Autodesk Inventor part; units mm, degrees
ref_plane "YZ Plane" through (0, 0, 0) normal (1, 0, 0) x (0, 1, 0)
ref_plane "XZ Plane" through (0, 0, 0) normal (0, 1, 0) x (-1, 0, 0)
ref_plane "XY Plane" through (0, 0, 0) normal (0, 0, 1) x (1, 0, 0)
sketch "T-Slot 4040 Base" plane through (0, 0, 0) normal (0, 0, 1) x (1, 0, 0)
  line L0 (-28, 0) -> (28, 0) construction
  line L1 (0, -28) -> (0, 28) construction
  circle A0 centre (0, 0) radius 5.1
  line L2 (-7.5, -7.5) -> (7.5, -7.5)
  line L3 (7.5, -7.5) -> (7.5, 7.5)
  line L4 (7.5, 7.5) -> (-7.5, 7.5)
  line L5 (-7.5, 7.5) -> (-7.5, -7.5)
  line L6 (-7.5, -7.5) -> (7.5, 7.5) construction
  line L7 (7.5, -7.5) -> (-7.5, 7.5) construction
  line L8 (-20, 20) -> (20, 20)
  line L9 (20, 20) -> (20, -20)
  line L10 (20, -20) -> (-20, -20)
  line L11 (-20, -20) -> (-20, 20)
  line L12 (-20, 20) -> (20, -20) construction
  line L13 (20, 20) -> (-20, -20) construction
  line L14 (20, 5) -> (14.5, 5)
  line L15 (14.5, 5) -> (14.5, 10)
  line L16 (14.5, 10) -> (12.4749, 10)
  line L17 (12.4749, 10) -> (7.5, 5.0251)
  line L18 (5, 20) -> (5, 14.5)
  line L19 (5, 14.5) -> (10, 14.5)
  line L20 (10, 14.5) -> (10, 12.4749)
  line L21 (10, 12.4749) -> (5.0251, 7.5)
  line L22 (18.5, 18.5) -> (11.5, 18.5)
  line L23 (11.5, 18.5) -> (11.5, 11.5)
  line L24 (11.5, 11.5) -> (18.5, 11.5)
  line L25 (18.5, 11.5) -> (18.5, 18.5)
  line L26 (18.5, 18.5) -> (11.5, 11.5) construction
  line L27 (11.5, 18.5) -> (18.5, 11.5) construction
  line L28 (3.0732, 1.3088) -> (4.38, 2.6125) construction
  line L29 (5.905, 4.1338) -> (4.1393, 5.9037)
  line L30 (4.1393, 5.9037) -> (2.6122, 4.3802)
  line L31 (1.3075, 3.0787) -> (3.0732, 1.3088) construction
  line L32 (3.0732, 1.3088) -> (4.1393, 5.9037) construction
  line L33 (5.905, 4.1338) -> (1.3075, 3.0787) construction
  line L34 (4.38, 2.6125) -> (5.905, 4.1338)
  line L35 (2.6122, 4.3802) -> (1.3075, 3.0787) construction
  line L36 (-20, 5) -> (-14.5, 5)
  line L37 (-14.5, 5) -> (-14.5, 10)
  line L38 (-14.5, 10) -> (-12.4749, 10)
  line L39 (-12.4749, 10) -> (-7.5, 5.0251)
  line L40 (-5, 20) -> (-5, 14.5)
  line L41 (-5, 14.5) -> (-10, 14.5)
  line L42 (-10, 14.5) -> (-10, 12.4749)
  line L43 (-10, 12.4749) -> (-5.0251, 7.5)
  line L44 (-18.5, 18.5) -> (-11.5, 18.5)
  line L45 (-11.5, 18.5) -> (-11.5, 11.5)
  line L46 (-11.5, 11.5) -> (-18.5, 11.5)
  line L47 (-18.5, 11.5) -> (-18.5, 18.5)
  line L48 (-5.905, 4.1338) -> (-4.1393, 5.9037)
  line L49 (-4.1393, 5.9037) -> (-2.6122, 4.3802)
  line L50 (-4.38, 2.6125) -> (-5.905, 4.1338)
  line L51 (7.5, -7.5) -> (-7.5, -7.5)
  line L52 (20, -5) -> (14.5, -5)
  line L53 (14.5, -5) -> (14.5, -10)
  line L54 (14.5, -10) -> (12.4749, -10)
  line L55 (12.4749, -10) -> (7.5, -5.0251)
  line L56 (5, -20) -> (5, -14.5)
  line L57 (5, -14.5) -> (10, -14.5)
  line L58 (10, -14.5) -> (10, -12.4749)
  line L59 (10, -12.4749) -> (5.0251, -7.5)
  line L60 (18.5, -18.5) -> (11.5, -18.5)
  line L61 (11.5, -18.5) -> (11.5, -11.5)
  line L62 (11.5, -11.5) -> (18.5, -11.5)
  line L63 (18.5, -11.5) -> (18.5, -18.5)
  line L64 (18.5, -18.5) -> (11.5, -11.5) construction
  line L65 (11.5, -18.5) -> (18.5, -11.5) construction
  line L66 (3.0732, -1.3088) -> (4.38, -2.6125) construction
  line L67 (5.905, -4.1338) -> (4.1393, -5.9037)
  line L68 (4.1393, -5.9037) -> (2.6122, -4.3802)
  line L69 (1.3075, -3.0787) -> (3.0732, -1.3088) construction
  line L70 (3.0732, -1.3088) -> (4.1393, -5.9037) construction
  line L71 (5.905, -4.1338) -> (1.3075, -3.0787) construction
  line L72 (4.38, -2.6125) -> (5.905, -4.1338)
  line L73 (2.6122, -4.3802) -> (1.3075, -3.0787) construction
  line L74 (-4.38, -2.6125) -> (-5.905, -4.1338)
  line L75 (-4.1393, -5.9037) -> (-2.6122, -4.3802)
  line L76 (-5.905, -4.1338) -> (-4.1393, -5.9037)
  line L77 (-12.4749, -10) -> (-7.5, -5.0251)
  line L78 (-10, -12.4749) -> (-5.0251, -7.5)
  line L79 (-10, -14.5) -> (-10, -12.4749)
  line L80 (-5, -14.5) -> (-10, -14.5)
  line L81 (-5, -20) -> (-5, -14.5)
  line L82 (-18.5, -18.5) -> (-11.5, -18.5)
  line L83 (-11.5, -18.5) -> (-11.5, -11.5)
  line L84 (-11.5, -11.5) -> (-18.5, -11.5)
  line L85 (-18.5, -11.5) -> (-18.5, -18.5)
  line L86 (-14.5, -10) -> (-12.4749, -10)
  line L87 (-14.5, -5) -> (-14.5, -10)
  line L88 (-20, -5) -> (-14.5, -5)
  point P0 (15, 15)
  point P1 (3.6062, 3.6062)
  point P2 (3.6062, 3.6062)
  point P3 (15, -15)
  point P4 (3.6062, -3.6062)
  point P5 (3.6062, -3.6062)
  dimension "d9" = 10.2
  dimension "d12" = 40
  dimension "d13" = 40
  dimension "d14" = 5.5
  dimension "d15" = 15
  dimension "d16" = 7
  dimension "d17" = 10
  dimension "d20" = 1.75
  dimension "d21" = 7
  dimension "d22" = 2
  dimension "d29" = 1.5
  dimension "d30" = 2.5
extrude "Extrusion1" add sketch "T-Slot 4040 Base" along normal blind 1500 contours L5 L4 L3 L2 | L2 L78 L79 L80 L81 L10 L11 L88 L87 L86 L77 L5 | L2 L3 L55 L54 L53 L52 L9 L10 L56 L57 L58 L59 | L39 L38 L37 L36 L11 L8 L40 L41 L42 L43 L4 L5 | L3 L4 L21 L20 L19 L18 L8 L9 L14 L15 L16 L17
fillet "Rundung1" radius 1 16 edges at (11.5, 18.5, 750) (18.5, 18.5, 750) (18.5, 11.5, 750) (11.5, 11.5, 750) (-11.5, 18.5, 750) (-18.5, 18.5, 750) (-18.5, 11.5, 750) (-11.5, 11.5, 750) (-18.5, -11.5, 750) (-11.5, -11.5, 750) (-11.5, -18.5, 750) (-18.5, -18.5, 750) (11.5, -18.5, 750) (11.5, -11.5, 750) (18.5, -11.5, 750) (18.5, -18.5, 750)
fillet "Rundung2" radius 3 4 edges at (20, 20, 750) (20, -20, 750) (-20, -20, 750) (-20, 20, 750)
properties part number "T-SLOT 4040 B-Type 1500mm"
Geometry check sheet. Reference: the model listing, model coordinates, mm. Give positions to 0.01 mm unless a question says otherwise; leave off trailing zeros.
(1) Thickness scan on L1, parallel to X at y = 17, z = 1359; L2, parallel to Y at x = 13.5, z = 735; L3, parallel to Y at x = 18, z = 530. Record the ranges inside material, lowest first.
From the geometry:
L1: x = -20 to -18.5, -11.5 to -5, 5 to 11.5, 18.5 to 20
L2: y = -20 to -18.5, -11.5 to -10, 10 to 11.5, 18.5 to 20
L3: y = -19.83 to -18.37, -11.63 to -5, 5 to 11.63, 18.37 to 19.83
(2) Section check A-A on z = 177.5. Count the separate pieces of the cut face and the enclosed holes in it, then the cut area to 3 significant figures.
From the geometry:
separate pieces: 1
enclosed holes: 5
area: 616 mm2
(3) Depth check by flat-ended pin: pin 1 Ø12 at (x, z) = (4.5, 991.5) entering from -Y; pin 2 Ø1 at (x, y) = (-2.5, -1) entering from +Z (3 decimals); pin 3 Ø2 at (x, z) = (-2, 1032) entering from -Y; pin 4 Ø3 at (y, z) = (0.5, 486.5) entering from +X. Enter the tip coordinate at first touch or a pass-through.
From the geometry:
pin 1: stops at y = -20
pin 2: passes through
pin 3: stops at y = -7.5
pin 4: stops at x = 7.5
